Check sheet for the modelled part. Datum: model origin and axes. Units: mm. A direction names the side the tool comes from. Coordinates: 2 decimals unless noted, no trailing zeros. Loops run counter-clockwise (first coordinate to the right, second up) from the corner with the lowest first, then second, coordinate; pieces in that order, holes last. Notation, with made-up numbers: M -10,75 L 1,75 A24 ccw 1,100 Z; hole C -37.5,-23 d4. An arc over 180 degrees is marked long. Return JSON: item names as keys, results as strings.
from build123d import *

# Parameters (mm, degrees)
F0_R     = 3
F0_R_2   = 1.5
F0_R_3   = 5
F1_DEPTH = 4


with BuildPart() as f1:
    # F0 (on Right) → F1 (new body)
    with BuildSketch(Plane.YZ):
        with BuildLine():
            Line((-2.213923, 9.815771), (-50.172412, 4.496696))
            ThreePointArc((-50.172412, 4.496696), (-54.497093, -0.161719), (-49.848975, -4.497465))
            Line((-49.848975, -4.497465), (-19.228159, -1.781642))
            Line((-19.228159, -1.781642), (-10.071731, -4.497465))
            Line((-10.071731, -4.497465), (-4.982847, -8.347222))
            Line((-4.982847, -8.347222), (-4.982847, -50.413808))
            ThreePointArc((-4.982847, -50.413808), (-0.389649, -54.984794), (4.858025, -51.183044))
            Line((4.858025, -51.183044), (4.987747, -49.650171))
            Line((4.987747, -49.650171), (8.680819, -6.010615))
            Line((8.680819, -6.010615), (9.067407, -1.442462))
            ThreePointArc((9.067407, -1.442462), (8.988122, -0.04027), (8.522012, 1.284557))
            Line((8.522012, 1.284557), (6.057092, 6.02837))
            ThreePointArc((6.057092, 6.02837), (4.881819, 7.512762), (3.238884, 8.453747))
            Line((3.238884, 8.453747), (-0.044164, 9.577011))
            ThreePointArc((-0.044164, 9.577011), (-1.115855, 9.816243), (-2.213923, 9.815771))
        make_face()
        with Locations((0, -50)):
            Circle(F0_R, mode=Mode.SUBTRACT)
        with Locations((-50, 0)):
            Circle(F0_R_2, mode=Mode.SUBTRACT)
        Circle(F0_R_3, mode=Mode.SUBTRACT)
        with BuildLine():
            Line((47.908556, 3.875873), (6.057092, 6.02837))
            Line((6.057092, 6.02837), (8.522012, 1.284557))
            ThreePointArc((8.522012, 1.284557), (8.988122, -0.04027), (9.067407, -1.442462))
            Line((9.067407, -1.442462), (8.680819, -6.010615))
            Line((8.680819, -6.010615), (47.908556, -1.356372))
            Line((47.908556, -1.356372), (47.908556, 3.875873))
        make_face()
        with BuildLine():
            Line((4.987747, -49.650171), (4.858025, -51.183044))
            ThreePointArc((4.858025, -51.183044), (4.982191, -50.421626), (4.987747, -49.650171))
        make_face()
    extrude(amount=F1_DEPTH)


solid = f1.part
1) Section check C-C on y = -7. Record the cut outline in (x, z).
Answers:
{"outline": "M 0,-6.82 L 4,-6.82 L 4,9.28 L 0,9.28 Z"}
2) Go/stop test with flat-tipped pins: pin 1 Ø1 at (x, z) = (1.5, -7) entering from +Y; pin 2 Ø2 at (x, z) = (1, -14.5) entering from -Y. Record where each tip stops, or that it passes through.
Answers:
{"pin 1": "y = 8.64", "pin 2": "y = -4.98"}
3) Set-up check for faces 5 (the face through (2, -4.983, -29)), 6 (the face through (1.97, -14.71, -3.12)), 7 (the face through (1.97, 6.81, -28.14)): record each of +Z, -Z, +X, -X, +Y, -Y from which the full face is reachable in a straight line by a thin tool's end or side.
Answers:
{"face 5": "-Z, +X, -X, -Y", "face 6": "-Z, +X, -X", "face 7": "-Z, +X, -X, +Y"}
4) Draft check along Z on faces 1 (the face through (1.97, -34.75, -3.16)), 2 (the face through (1.972, -25.857, 7.193)), 3 (the face through (2, 0, -47)), 4 (the face through (1.97, -51.5, 0.07)). Enter one of: +Z half, -Z half, draft (parallel to the pull), parting line (faces both ways), or undercut.
Answers:
{"face 1": "-Z half", "face 2": "+Z half", "face 3": "undercut", "face 4": "undercut"}
5) Section check A-A on z = 0. Record the cut outline in (x, y).
Answers:
{"outline": "M 0,-54.5 L 4,-54.5 L 4,-51.5 L 0,-51.5 Z; M 0,-48.5 L 4,-48.5 L 4,-5 L 0,-5 Z; M 0,5 L 4,5 L 4,47.91 L 0,47.91 Z"}
6) Section check D-D on z = -32. Record the cut outline in (x, y), then the cut area to 3 significant figures.
Answers:
{"outline": "M 0,-4.98 L 4,-4.98 L 4,6.48 L 0,6.48 Z", "area": "45.9 mm²"}
7) Scan lines: line 1 along Z through (x, y) = (0.8, 0); line 2 along Z through (x, y) = (2.8, -50); line 3 along Z through (x, y) = (2.5, 4.5). Record each from-to range of solid material in increasing order. Write a range as [from, to].
Answers:
{"line 1": "[-55, -53], [-47, -5], [5, 9.56]", "line 2": "[-4.5, -1.5], [1.5, 4.52]", "line 3": "[-52.18, -2.18], [2.18, 7.81]"}
8) Section check B-B on x = 1. Record the cut outline in (y, z), then the cut area to 3 significant figures.
Answers:
{"outline": "M -50.17,4.5 A4.5 ccw -49.85,-4.5 L -19.23,-1.78 L -10.07,-4.5 L -4.98,-8.35 L -4.98,-50.41 A5 ccw 4.86,-51.18 A5 ccw 4.99,-49.65 L 8.68,-6.01 L 47.91,-1.36 L 47.91,3.88 L 6.06,6.03 A5 ccw 3.24,8.45 L -0.04,9.58 A5 ccw -2.21,9.82 Z; hole C -50,0 d3; hole C 0,0 d10; hole C 0,-50 d6", "area": "1,480 mm²"}
